from build123d import *

# Parameters (mm, degrees)
F0_W      = 210
F0_H      = 30
F0_W_2    = 110
F0_H_2    = 14
F1_DEPTH  = 5
F2_R      = 10.6
F2_R_2    = 1
F2_R_3    = 4.5
F2_W      = 43
F2_H      = 22
F2_R_4    = 2.75
F3_DEPTH  = 3
F4_DEPTH  = 25
F5_R      = 14.99999
F6_R      = 6.99999
F7_R      = 1
F8_DEPTH  = 25
F9_W      = 5
F9_H      = 8
F10_DEPTH = 8
F11_W     = 5.5
F11_H     = 5.5
F12_DEPTH = 6
F13_W     = 5.5
F13_H     = 5.5
F14_DEPTH = 6
F15_W     = 5.5
F15_H     = 5.5
F16_W     = 5.5
F16_H     = 5.5
F17_DEPTH = 6
F9_W_2    = 45
F9_H_2    = 2.5
F18_DEPTH = 8
F19_DEPTH = 0.5
F20_R     = 1.5


# Not quite as in the source:
# - a fillet or chamfer is up to 0.001 mm smaller than in the source, because OpenCascade refuses the exact size
# - a feature names something its author has since deleted; it is built from what else it names


with BuildPart() as f1:
    # F0 (on Top) → F1 (new body)
    with BuildSketch(Plane.XY):
        with Locations((-5, -11.8972941886)):
            Rectangle(F0_W, F0_H)
        with Locations((15, -11.8972941886)):
            Rectangle(F0_W_2, F0_H_2, mode=Mode.SUBTRACT)
    extrude(amount=F1_DEPTH)

    # F2 (on face) → F3 (cut)
    with BuildSketch(Plane.XY.offset(5)):
        with Locations((85, -11.8972941886)):
            Circle(F2_R)
        with Locations((85, -19.3972941886)):
            Circle(F2_R_2, mode=Mode.SUBTRACT)
        with Locations((85, -11.8972941886)):
            Circle(F2_R_3, mode=Mode.SUBTRACT)
        with Locations((77.5, -11.8972941886)):
            Circle(F2_R_2, mode=Mode.SUBTRACT)
        with Locations((92.5, -11.8972941886)):
            Circle(F2_R_2, mode=Mode.SUBTRACT)
        with Locations((85, -4.3972941886)):
            Circle(F2_R_2, mode=Mode.SUBTRACT)
        with Locations((-75.5, -11.8972941886)):
            Rectangle(F2_W, F2_H)
        with Locations((-65, -11.8972941886)):
            Circle(F2_R_4, mode=Mode.SUBTRACT)
    extrude(amount=-F3_DEPTH, mode=Mode.SUBTRACT)

    # F2 (on face) → F4 (cut)
    with BuildSketch(Plane.XY.offset(5)):
        with Locations((-75.5, -11.8972941886)):
            Rectangle(F2_W, F2_H)
        with Locations((-65, -11.8972941886)):
            Circle(F2_R_4, mode=Mode.SUBTRACT)
        with Locations((85, -11.8972941886)):
            Circle(F2_R_3)
        with Locations((-65, -11.8972941886)):
            Circle(F2_R_4)
        with Locations((85, -4.3972941886)):
            Circle(F2_R_2)
        with Locations((77.5, -11.8972941886)):
            Circle(F2_R_2)
        with Locations((85, -19.3972941886)):
            Circle(F2_R_2)
        with Locations((92.5, -11.8972941886)):
            Circle(F2_R_2)
    extrude(amount=-F4_DEPTH, mode=Mode.SUBTRACT)

    # F5 (radius 15 in the source; OpenCascade refuses exactly that, so slightly less here)
    f5_edges = [f1.edges().sort_by_distance(p)[0] for p in [
        (100, 3.102706, 2.5),
        (100, -26.897294, 2.5),
        (-110, -26.897294, 2.5),
        (-110, 3.102706, 2.5),
    ]]
    fillet(f5_edges, radius=F5_R)

    # F6 (radius 7 in the source; OpenCascade refuses exactly that, so slightly less here)
    f6_edges = [f1.edges().sort_by_distance(p)[0] for p in [
        (-40, -4.897294, 2.5),
        (-40, -18.897294, 2.5),
        (70, -4.897294, 2.5),
        (70, -18.897294, 2.5),
    ]]
    fillet(f6_edges, radius=F6_R)

    # F7
    f7_edges = [f1.edges().sort_by_distance(p)[0] for p in [
        (-97, -0.897294, 2.5),
        (-97, -22.897294, 2.5),
        (-54, -0.897294, 2.5),
        (-54, -22.897294, 2.5),
    ]]
    fillet(f7_edges, radius=F7_R)

    # F2 (on face) → F8 (cut)
    with BuildSketch(Plane.XY.offset(5)):
        with Locations((-100, -6.8972941886)):
            Circle(F2_R_2)
        with Locations((-100, -16.8972941886)):
            Circle(F2_R_2)
        with Locations((-51, -6.8972941886)):
            Circle(F2_R_2)
        with Locations((-51, -16.8972941886)):
            Circle(F2_R_2)
    extrude(amount=-F8_DEPTH, mode=Mode.SUBTRACT)

    # F9 (on face) → F10 (join)
    with BuildSketch(Plane.XY.offset(5)):
        with Locations((-27.5, -0.8972941886)):
            Rectangle(F9_W, F9_H)
        Polygon((-10, 3.1027058114), (-15, 3.1027058114), (-15, -4.8972941886), (-10, -4.8972941886), (-10, -2.3972941886), align=None)
        Polygon((40, 3.1027058114), (35, 3.1027058114), (35, -2.3972941886), (35, -4.8972941886), (40, -4.8972941886), align=None)
        with Locations((47.5, -0.8972941886)):
            Rectangle(F9_W, F9_H)
    extrude(amount=F10_DEPTH)

    # F11 (on face) → F12 (cut)
    with BuildSketch(Plane(origin=(-30, 0, 0), x_dir=(0, -1, 0), z_dir=(-1, 0, 0))):
        with Locations((2.1472941886, 8.25)):
            Rectangle(F11_W, F11_H)
    extrude(amount=-F12_DEPTH, mode=Mode.SUBTRACT)

    # F13 (on face) → F14 (cut)
    with BuildSketch(Plane(origin=(-15, 0, 0), x_dir=(0, -1, 0), z_dir=(-1, 0, 0))):
        with Locations((-0.3527058114, 8.25)):
            Rectangle(F13_W, F13_H)
    extrude(amount=-F14_DEPTH, mode=Mode.SUBTRACT)

    # F15 (on face) + F16 (on face) → F17 (cut)
    with BuildSketch(Plane(origin=(35, 0, 0), x_dir=(0, -1, 0), z_dir=(-1, 0, 0))):
        with Locations((-0.3527058114, 8.25)):
            Rectangle(F15_W, F15_H)
    with BuildSketch(Plane(origin=(45, 0, 0), x_dir=(0, -1, 0), z_dir=(-1, 0, 0))):
        with Locations((2.1472941886, 8.25)):
            Rectangle(F16_W, F16_H)
    extrude(amount=-F17_DEPTH, mode=Mode.SUBTRACT)

    # F9 (on face) → F18 (join)
    with BuildSketch(Plane.XY.offset(5)):
        with Locations((12.5, -3.6472941886)):
            Rectangle(F9_W_2, F9_H_2)
    extrude(amount=F18_DEPTH)

    # F19 (cut): faces of the model
    f19_faces = [f1.faces().sort_by_distance(p)[0] for p in [
        (37.5, 3.1027058114, 12),
        (-12.5, 3.1027058114, 12),
        (47.5, -4.8972941886, 12),
        (-27.5, -4.8972941886, 12),
    ]]
    extrude(f19_faces, amount=-F19_DEPTH, dir=(0, 1, 0), mode=Mode.SUBTRACT)

    # F20
    f20_edges = [f1.edges().sort_by_distance(p)[0] for p in [
        (-27.5, 3.102706, 13),
        (-27.5, -4.897294, 13),
        (12.5, -4.897294, 13),
        (-12.5, 2.602706, 13),
        (-12.5, -2.397294, 5.5),
        (-12.5, -2.397294, 11),
        (-27.5, 0.602706, 5.5),
        (-27.5, 0.602706, 11),
        (37.5, 2.602706, 13),
        (47.5, 3.102706, 13),
        (47.5, -4.897294, 13),
        (37.5, -2.397294, 11),
        (37.5, -2.397294, 5.5),
        (47.5, 0.602706, 5.5),
        (47.5, 0.602706, 11),
    ]]
    fillet(f20_edges, radius=F20_R)


solid = f1.part
Can you work these out from the model? Positions are in its coordinate system, mm. A direction names the side the tool comes from. Coordinates: 2 decimals unless noted, no trailing zeros. Loops run counter-clockwise (first coordinate to the right, second up) from the corner with the lowest first, then second, coordinate; pieces in that order, holes last. Notation, with made-up numbers: (54.25, 8) - (70.25, 8) arc R18 cw to (70.25, 27) - close; hole circle Ø11 at (41.25, 67). An arc over 180 degrees is marked (long way). Answer as a JSON object with one key per item and string values. Group by question number.
Item 1: If we mould it in two halves opening along Y, with no side actions, what happens to faces 1 (the face through (-6, 3.103, 3)), 2 (the face through (14, -18.897, 2)), 3 (the face through (-15, -3, 9)), 4 (the face through (-76, -0.897, 3))? For each: released by +Y, released by -Y, zero draft, split by the parting line, or undercut.
Item 2: For pin 1 (2.5 mm diameter, centred on x = -19.5, y = 0, fed in from +Z); pin 2 (3 mm diameter, centred on x = 77.5, y = -11.9, fed in from +Z); pin 3 (1.6 mm diameter, centred on y = -1, z = 5.5, fed in from +X), each with a flat end and sliding along its axis, tell me the tip position at first contact or that it passes through.
Item 3: If I drill on L1, parallel to X at y = 1.5, z = 5.25; L2, parallel to Y at x = -51, z = 1.45; L3, parallel to X at y = -21, z = 3.75, over which ranges is the centre line in solid material (lowest first)? Write a range as from..to.
Item 4: If we section it at A-A (x = 54): List the corners of the cut face in (y, z) for me.
Item 5: On a 3-axis mill with a long thin cutter (end or side, diameter ignored), from which of +Z, -Z, +X, -X, +Y, -Y can I reach the whole of each face in a straight line? I mean faces 5 (the face through (42, -1, 5)), 6 (the face through (-28, -3, 11)), 7 (the face through (68, -7, 3)). Say none if no direction works.
Returned:
{
 "1": {"face 1": "released by +Y", "face 2": "undercut", "face 3": "zero draft", "face 4": "undercut"},
 "2": {"pin 1": "stops at z = 5", "pin 2": "stops at z = 2", "pin 3": "stops at x = 95.93"},
 "3": {"L1": "x = -30..-25, -15..-10, 35..40, 45..50", "L2": "y = -26.9..-17.9, -15.9..-7.9, -5.9..3.1", "L3": "x = -106.92..-97, -54..79.57, 90.43..96.92"},
 "4": {"outline": "(-26.9, 0) - (-18.9, 0) - (-18.9, 5) - (-26.9, 5) - close; (-4.9, 0) - (3.1, 0) - (3.1, 5) - (-4.9, 5) - close"},
 "5": {"face 5": "+Z, +Y, -Y", "face 6": "-X, -Y", "face 7": "+Z, -Z"}
}
